```python
from build123d import *

# Parameters (mm, degrees)
BOSS_EXTRUDE1_DEPTH = 3
FILLET1_R           = 60
FILLET2_R           = 8
SKETCH3_R           = 1.45
SKETCH3_R_2         = 5.6
SKETCH3_W           = 9.2
SKETCH3_H           = 7.5
CUT_EXTRUDE1_DEPTH  = 125.676613305
SKETCH4_R           = 1.5
SKETCH4_W           = 8
SKETCH4_H           = 5
CUT_EXTRUDE2_DEPTH  = 125.676613305
SKETCH5_W           = 5
SKETCH5_H           = 8
CUT_EXTRUDE3_DEPTH  = 125.676613305
FILLET3_R           = 9
SKETCH6_R           = 1.5
SKETCH6_W           = 5
SKETCH6_H           = 6
CUT_EXTRUDE4_DEPTH  = 125.676613305


with BuildPart() as part:
    # Sketch1 → Boss-Extrude1 (new body)
    with BuildSketch(Plane.XY):
        Polygon((-83.391188804, -3.05320323), (-63.103878976, 32.08544814), (-12.25, 32.08544814), (-12.25, -8), (12.25, -8), (12.25, 32.08544814), (63.103878976, 32.08544814), (83.391188804, -3.05320323), (104.608811196, 9.19679677), (91.394042166, 32.08544814), (91.394042166, 72.08544814), (-91.394042166, 72.08544814), (-91.394042166, 32.08544814), (-104.608811196, 9.19679677), align=None)
        with BuildLine():
            ThreePointArc((-72.410784769, 15.965414445), (-60.610101085, 27.766098129), (-44.49006739, 32.08544814))
            Line((-44.49006739, 32.08544814), (-63.103878976, 32.08544814))
            Line((-63.103878976, 32.08544814), (-72.410784769, 15.965414445))
        make_face()
        with BuildLine():
            Line((-12.25, -0.15461925), (-12.25, 32.08544814))
            Line((-12.25, 32.08544814), (-44.49006739, 32.08544814))
            ThreePointArc((-44.49006739, 32.08544814), (-21.692897113, 22.642551027), (-12.25, -0.15461925))
        make_face()
        with BuildLine():
            Line((12.25, 32.08544814), (12.25, -0.15461925))
            ThreePointArc((12.25, -0.15461925), (21.692897113, 22.642551027), (44.49006739, 32.08544814))
            Line((44.49006739, 32.08544814), (12.25, 32.08544814))
        make_face()
        with BuildLine():
            Line((63.103878976, 32.08544814), (44.49006739, 32.08544814))
            ThreePointArc((44.49006739, 32.08544814), (60.610101085, 27.766098129), (72.410784769, 15.965414445))
            Line((72.410784769, 15.965414445), (63.103878976, 32.08544814))
        make_face()
    extrude(amount=BOSS_EXTRUDE1_DEPTH)

    # Fillet1
    fillet1_edges = [part.edges().sort_by_distance(p)[0] for p in [
        (-91.394042166, 32.08544814, 1.5),
        (91.394042166, 32.08544814, 1.5),
    ]]
    fillet(fillet1_edges, radius=FILLET1_R)

    # Fillet2
    fillet2_edges = [part.edges().sort_by_distance(p)[0] for p in [
        (-104.608811196, 9.19679677, 1.5),
        (-83.391188804, -3.05320323, 1.5),
        (-12.25, -8, 1.5),
        (12.25, -8, 1.5),
        (83.391188804, -3.05320323, 1.5),
        (104.608811196, 9.19679677, 1.5),
    ]]
    fillet(fillet2_edges, radius=FILLET2_R)

    # Sketch3 → Cut-Extrude1 (cut, through all)
    with BuildSketch(Plane.XY.offset(3)):
        with Locations((87.596023553, 31.763809346)):
            Circle(SKETCH3_R)
        with Locations((72.353976447, 22.963809346)):
            Circle(SKETCH3_R)
        with Locations((8.8, 20.05)):
            Circle(SKETCH3_R)
        with Locations((-8.8, 20.05)):
            Circle(SKETCH3_R)
        with Locations((-87.596023553, 31.763809346)):
            Circle(SKETCH3_R)
        with Locations((-72.353976447, 22.963809346)):
            Circle(SKETCH3_R)
        Circle(SKETCH3_R_2)
        with Locations((-90, 10)):
            Circle(SKETCH3_R_2)
        with Locations((90, 10)):
            Circle(SKETCH3_R_2)
        with BuildLine():
            Line((-53.35839931, 57.665114066), (-55.45839931, 54.02780737))
            Line((-55.45839931, 54.02780737), (-52.340707856, 52.22780737))
            ThreePointArc((-52.340707856, 52.22780737), (-51.657770716, 52.137896989), (-51.111284993, 52.557230233))
            Line((-51.111284993, 52.557230233), (-49.911284993, 54.635691202))
            ThreePointArc((-49.911284993, 54.635691202), (-49.821374613, 55.318628343), (-50.240707856, 55.865114066))
            Line((-50.240707856, 55.865114066), (-53.35839931, 57.665114066))
        make_face()
        with BuildLine():
            Line((7.9, 59.6), (7.9, 55.4))
            Line((7.9, 55.4), (11.5, 55.4))
            ThreePointArc((11.5, 55.4), (12.136396103, 55.663603897), (12.4, 56.3))
            Line((12.4, 56.3), (12.4, 58.7))
            ThreePointArc((12.4, 58.7), (12.136396103, 59.336396103), (11.5, 59.6))
            Line((11.5, 59.6), (7.9, 59.6))
        make_face()
        with BuildLine():
            Line((67.04160069, 65.565114066), (69.14160069, 61.92780737))
            Line((69.14160069, 61.92780737), (72.259292144, 63.72780737))
            ThreePointArc((72.259292144, 63.72780737), (72.678625387, 64.274293092), (72.588715007, 64.957230233))
            Line((72.588715007, 64.957230233), (71.388715007, 67.035691202))
            ThreePointArc((71.388715007, 67.035691202), (70.842229284, 67.455024446), (70.159292144, 67.365114066))
            Line((70.159292144, 67.365114066), (67.04160069, 65.565114066))
        make_face()
        Polygon((-68.766283143, 37.577876431), (-76.733716857, 42.177876431), (-80.483716857, 35.682685902), (-72.516283143, 31.082685902), align=None)
        with Locations((0, 30.75)):
            Rectangle(SKETCH3_W, SKETCH3_H)
        Polygon((76.733716857, 42.177876431), (68.766283143, 37.577876431), (72.516283143, 31.082685902), (80.483716857, 35.682685902), align=None)
    extrude(amount=-CUT_EXTRUDE1_DEPTH, mode=Mode.SUBTRACT)

    # Sketch4 → Cut-Extrude2 (cut, through all)
    with BuildSketch(Plane.XY.offset(3)):
        with Locations((-31.394042166, 59.58544814)):
            Circle(SKETCH4_R)
        with Locations((31.394042166, 59.58544814)):
            Circle(SKETCH4_R)
        with Locations((-85.894042166, 59.58544814)):
            Circle(SKETCH4_R)
        with Locations((85.894042166, 59.58544814)):
            Circle(SKETCH4_R)
        with Locations((-42.394042166, 59.58544814)):
            Rectangle(SKETCH4_W, SKETCH4_H)
        with Locations((-20.394042166, 59.58544814)):
            Rectangle(SKETCH4_W, SKETCH4_H)
        with Locations((20.394042166, 59.58544814)):
            Rectangle(SKETCH4_W, SKETCH4_H)
        with Locations((42.394042166, 59.58544814)):
            Rectangle(SKETCH4_W, SKETCH4_H)
    extrude(amount=-CUT_EXTRUDE2_DEPTH, mode=Mode.SUBTRACT)

    # Sketch5 → Cut-Extrude3 (cut, through all)
    with BuildSketch(Plane.XY.offset(3)):
        with Locations((-85.894042166, 50.08544814)):
            Rectangle(SKETCH5_W, SKETCH5_H)
        with Locations((85.894042166, 50.08544814)):
            Rectangle(SKETCH5_W, SKETCH5_H)
    extrude(amount=-CUT_EXTRUDE3_DEPTH, mode=Mode.SUBTRACT)

    # Fillet3
    fillet3_edges = [part.edges().sort_by_distance(p)[0] for p in [
        (-91.394042166, 72.08544814, 1.5),
        (91.394042166, 72.08544814, 1.5),
    ]]
    fillet(fillet3_edges, radius=FILLET3_R)

    # Sketch6 → Cut-Extrude4 (cut, through all)
    with BuildSketch(Plane.XY.offset(3)):
        with Locations((-31.394042166, 46.08544814)):
            Circle(SKETCH6_R)
        with Locations((31.394042166, 46.08544814)):
            Circle(SKETCH6_R)
        with Locations((31.394042166, 38.08544814)):
            Rectangle(SKETCH6_W, SKETCH6_H)
        with Locations((31.394042166, 54.08544814)):
            Rectangle(SKETCH6_W, SKETCH6_H)
        with Locations((-31.394042166, 54.08544814)):
            Rectangle(SKETCH6_W, SKETCH6_H)
        with Locations((-31.394042166, 38.08544814)):
            Rectangle(SKETCH6_W, SKETCH6_H)
    extrude(amount=-CUT_EXTRUDE4_DEPTH, mode=Mode.SUBTRACT)


solid = part.part
```
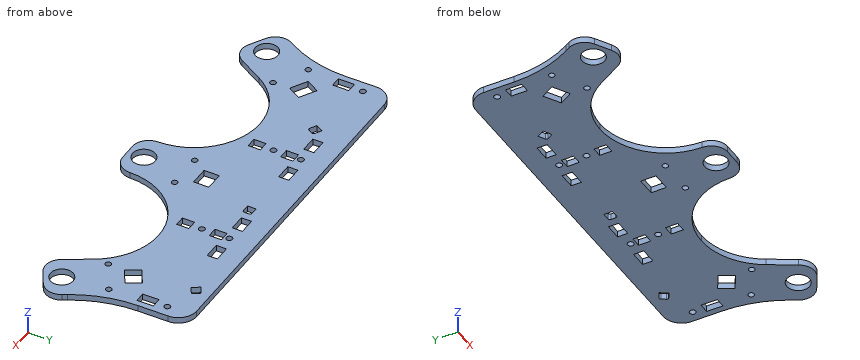
Read the model definition and answer for the solid it produces. Units are mm, in the model's axes. Give positions to 0.01 mm unless a question says otherwise; leave off trailing zeros. Write each loop counter-clockwise with the first axis right and the second up, starting at its lowest first coordinate (ties: lowest second). Pieces come first, ordered by that corner, then holes. Notation, with made-up numbers: (70.25, 0.25) - (111.25, 0.25) arc R7 ccw to (111.25, 10.25) - close; hole circle Ø2 at (-23, -2.75). An arc over 180 degrees is marked (long way). Write item = value, one per line. Start each with the question number.
Item 1: Find section D-D (x = 52.5). Give the vertices of the cut face in (y, z).
Item 2: Find section A-A (x = 0). Give the vertices of the cut face in (y, z).
Item 3: Find section C-C (x = -61.5). Give the vertices of the cut face in (y, z).
Item 4: Find the intervals of material crossed by probe 1 along X at (y, z) = (58, 0.85); probe 2 along X at (y, z) = (20, 0.7); probe 3 along X at (y, z) = (17.5, 0.7), in increasing order. Write a range as [from, to].
Item 5: Find section B-B (z = 1.6). State how many separate pieces and enclosed holes the cut face has, then the cut area to 3 significant figures.
Item 6: Each of these flat-tipped pins is pushed along its axis until it touches: P1, Ø1.5, axis at x = 9.5, z = 1.5, coming from the -Y side; P2, Ø1.5, axis at x = -40.5, z = 2, coming from the -Y side; P3, Ø1.5, axis at y = 40, z = 1.5, coming from the +X side. Where does it stop, or does it pass through?
Response:
q1.outline = (31.07, 0) - (72.09, 0) - (72.09, 3) - (31.07, 3) - close
q2.outline = (-8, 0) - (-5.6, 0) - (-5.6, 3) - (-8, 3) - close; (5.6, 0) - (27, 0) - (27, 3) - (5.6, 3) - close; (34.5, 0) - (72.09, 0) - (72.09, 3) - (34.5, 3) - close
q3.outline = (27.23, 0) - (72.09, 0) - (72.09, 3) - (27.23, 3) - close
q4.probe_1 = [-91.39, -46.39], [-38.39, -24.39], [-16.39, 7.9], [12.4, 16.39], [24.39, 38.39], [46.39, 91.39]
q4.probe_2 = [-98.41, -69.65], [-19.33, -10.25], [-7.35, 7.35], [10.25, 19.33], [69.65, 98.41]
q4.probe_3 = [-99.81, -71.47], [-17.51, 17.51], [71.47, 99.81]
q5.separate_pieces = 1
q5.enclosed_holes = 31
q5.area = 9,420 mm²
q6.P1 = -6.61
q6.P2 = 31.74
q6.P3 = 92.06
